Design review of the part built by this model. Coordinates are the model's own, in mm. A direction names the side the tool comes from. Round coordinates to 2 decimals unless told otherwise and drop trailing zeros. Write each loop counter-clockwise with the first axis right and the second up, starting at its lowest first coordinate (ties: lowest second). Pieces come first, ordered by that corner, then holes.
from build123d import *

# Parameters (mm, degrees)
SKETCH1_W               = 77.793311879
SKETCH1_H               = 102.364407774
SKETCH1_R               = 2.75
SKETCH1_R_2             = 2
SKETCH1_R_3             = 7.5
BOSS_EXTRUDE1_DEPTH     = 3
CUT_EXTRUDE1_DEPTH      = 69.323346558
CUT_EXTRUDE1_DEPTH_BACK = 69.323346558
SKETCH2_R               = 1.5
CUT_EXTRUDE2_DEPTH      = 69.323346558
CUT_EXTRUDE2_DEPTH_BACK = 69.323346558
SKETCH3_W               = 36
SKETCH3_H               = 12
SKETCH3_W_2             = 21
SKETCH3_H_2             = 3
SKETCH3_W_3             = 15
SKETCH3_H_3             = 5
SKETCH3_R               = 1.5
CUT_EXTRUDE3_DEPTH      = 69.323346558
CUT_EXTRUDE3_DEPTH_BACK = 69.323346558
SKETCH4_R               = 1.5
CUT_EXTRUDE4_DEPTH      = 69.323346558
CUT_EXTRUDE4_DEPTH_BACK = 69.323346558
SKETCH5_R               = 1.6
FILLET1_R               = 30
CUT_EXTRUDE5_DEPTH      = 69.323346558
CUT_EXTRUDE5_DEPTH_BACK = 69.323346558
SKETCH6_R               = 1.5


with BuildPart() as part:
    # Sketch1 → Boss-Extrude1 (new body)
    with BuildSketch(Plane(origin=(0, 0, 0), x_dir=(1, 0, 0), z_dir=(0, 1, 0))):
        with Locations((2.136088924, -3.364964086)):
            Rectangle(SKETCH1_W, SKETCH1_H)
        with Locations(Location((-16, 25, 0), (0, 0, 270))):
            Circle(SKETCH1_R, mode=Mode.SUBTRACT)
        with Locations(Location((16, 25, 0), (0, 0, 270))):
            Circle(SKETCH1_R, mode=Mode.SUBTRACT)
        with Locations(Location((-15, -25, 0), (0, 0, 270))):
            Circle(SKETCH1_R_2, mode=Mode.SUBTRACT)
        with Locations(Location((0, 0, 0), (0, 0, 270))):
            Circle(SKETCH1_R_3, mode=Mode.SUBTRACT)
        with Locations(Location((0, -40, 0), (0, 0, 270))):
            Circle(SKETCH1_R_2, mode=Mode.SUBTRACT)
    extrude(amount=BOSS_EXTRUDE1_DEPTH)

    # Sketch2 → Cut-Extrude1 (cut, two sides: drawn at the far end of the back side and taken through both)
    with BuildSketch(Plane(origin=(0, 3, 0), x_dir=(1, 0, 0), z_dir=(0, 1, 0)).offset(-CUT_EXTRUDE1_DEPTH_BACK)):
        with Locations(Location((7.5, -32.905563019, 0), (0, 0, 270))):
            Circle(SKETCH2_R)
        with Locations(Location((-7.5, -32.905563019, 0), (0, 0, 270))):
            Circle(SKETCH2_R)
        with Locations(Location((-32.2470535, 9.957590981, 0), (0, 0, 270))):
            Circle(SKETCH2_R)
        with Locations(Location((-24.7470535, 22.947972038, 0), (0, 0, 270))):
            Circle(SKETCH2_R)
        with Locations(Location((24.7470535, 22.947972038, 0), (0, 0, 270))):
            Circle(SKETCH2_R)
        with Locations(Location((32.2470535, 9.957590981, 0), (0, 0, 270))):
            Circle(SKETCH2_R)
    extrude(amount=CUT_EXTRUDE1_DEPTH + CUT_EXTRUDE1_DEPTH_BACK, mode=Mode.SUBTRACT)

    # Sketch3 → Cut-Extrude2 (cut, two sides: drawn at the far end of the back side and taken through both)
    with BuildSketch(Plane(origin=(0, 3, 0), x_dir=(1, 0, 0), z_dir=(0, 1, 0)).offset(-CUT_EXTRUDE2_DEPTH_BACK)):
        with Locations((18.5, 0)):
            Rectangle(SKETCH3_W, SKETCH3_H)
        with Locations((18.5, -20.5)):
            Rectangle(SKETCH3_W_2, SKETCH3_H_2)
        with Locations((19.434564823, -47)):
            Rectangle(SKETCH3_W_3, SKETCH3_H_3)
        with Locations(Location((38.5, -13.251338354, 0), (0, 0, 270))):
            Circle(SKETCH3_R)
        with Locations(Location((-1.5, -13.251338354, 0), (0, 0, 270))):
            Circle(SKETCH3_R)
    extrude(amount=CUT_EXTRUDE2_DEPTH + CUT_EXTRUDE2_DEPTH_BACK, mode=Mode.SUBTRACT)

    # Sketch4 → Cut-Extrude3 (cut, two sides: drawn at the far end of the back side and taken through both)
    with BuildSketch(Plane(origin=(0, 3, 0), x_dir=(1, 0, 0), z_dir=(0, 1, 0)).offset(-CUT_EXTRUDE3_DEPTH_BACK)):
        with Locations(Location((-11, 9, 0), (0, 0, 270))):
            Circle(SKETCH4_R)
        with Locations(Location((-11, -9, 0), (0, 0, 270))):
            Circle(SKETCH4_R)
    extrude(amount=CUT_EXTRUDE3_DEPTH + CUT_EXTRUDE3_DEPTH_BACK, mode=Mode.SUBTRACT)

    # Sketch5 → Cut-Extrude4 (cut, two sides: drawn at the far end of the back side and taken through both)
    with BuildSketch(Plane(origin=(0, 3, 0), x_dir=(1, 0, 0), z_dir=(0, 1, 0)).offset(-CUT_EXTRUDE4_DEPTH_BACK)):
        with Locations(Location((18.5, 38.28654225, 0), (0, 0, 270))):
            Circle(SKETCH5_R)
        with Locations(Location((-18.5, 38.28654225, 0), (0, 0, 270))):
            Circle(SKETCH5_R)
    extrude(amount=CUT_EXTRUDE4_DEPTH + CUT_EXTRUDE4_DEPTH_BACK, mode=Mode.SUBTRACT)

    # Fillet1
    fillet1_edges = [part.edges().sort_by_distance(p)[0] for p in [
        (-36.760567016, 1.5, -47.817239801),
        (41.032744863, 1.5, -47.817239801),
        (41.032744863, 1.5, 54.547167973),
        (-36.760567016, 1.5, 54.547167973),
    ]]
    fillet(fillet1_edges, radius=FILLET1_R)

    # Sketch6 → Cut-Extrude5 (cut, two sides: drawn at the far end of the back side and taken through both)
    with BuildSketch(Plane(origin=(0, 3, 0), x_dir=(1, 0, 0), z_dir=(0, 1, 0)).offset(-CUT_EXTRUDE5_DEPTH_BACK)):
        with Locations(Location((-17.49999993, 12.5, 0), (0, 0, 270))):
            Circle(SKETCH6_R)
        with Locations(Location((-17.49999993, -12.5, 0), (0, 0, 270))):
            Circle(SKETCH6_R)
    extrude(amount=CUT_EXTRUDE5_DEPTH + CUT_EXTRUDE5_DEPTH_BACK, mode=Mode.SUBTRACT)


solid = part.part
1) Add section A-A on z = 9. State the section outline as (x, y) points, and give its area (3 significant figures).
2) For P1, Ø0.9, axis at x = 14.5, y = 2, coming from the +Z side, flat-tipped, find the tip position at first contact; note if it passes through.
3) The part is to be moulded in two halves that separate along X. For faces 3 (the face through (19.581, 1.479, -39.466)), 4 (the face through (32.011, 1.521, -39.262)), 5 (the face through (2, 1, -47.817)), say which applies: pulls with the +X half, pulls with the -X half, needs draft (parallel to the pull), parting line crosses it, or undercut.
4) For line 1 along Z through (x, y) = (11.5, 0.65); line 2 along X through (y, z) = (2.8, -9); line 3 along X through (y, z) = (2.25, 32), list the stretches that pass through material, from the lowest coordinate up.
5) Add section B-B on y = 2.25. Count the separate pieces of the cut face and the enclosed holes in it, and give its area (3 significant figures).
6) For faces 1 (the face through (2, 1, 54.547)), 2 (the face through (11.935, 1, 47)), list the 3-axis set-ups (+Z, -Z, +X, -X, +Y, -Y) from which the entire face can be reached by the end or side of a thin tool; tool diameter is ignored.
Computed:
1. outline: (-36.76, 0) - (-12.5, 0) - (-12.5, 3) - (-36.76, 3) - close; (-9.5, 0) - (41.03, 0) - (41.03, 3) - (-9.5, 3) - close
1. area: 224 mm2
2. P1: stops at z = 54.4
3. face 3: undercut
3. face 4: pulls with the +X half
3. face 5: needs draft
4. line 1: z = -47.81 to -6, 6 to 19, 22 to 54.54
4. line 2: x = -36.76 to -33.4, -31.09 to -12.5, -9.5 to 31.09, 33.4 to 41.03
4. line 3: x = -35.82 to -8.7, -6.3 to 6.3, 8.7 to 40.09
5. separate pieces: 1
5. enclosed holes: 21
5. area: 6,340 mm2
6. face 1: +Z, +X, -X, +Y, -Y
6. face 2: +Y, -Y
